Autodesk Fusion 360 part; units mm, degrees
sketch "Sketch3" plane through (0, 0, 0) normal (0, 0, 1) x (1, 0, 0)
  line L0 (10, 15) -> (-10, 15)
  line L1 (-10, 15) -> (-10, -15)
  line L2 (-10, -15) -> (10, -15)
  line L3 (10, -15) -> (10, 15)
  line L4 (10, 15) -> (-10, -15) construction
  line L5 (-10, 15) -> (10, -15) construction
  circle A0 centre (-5.1854, -3.7051) radius 3.5
  circle A1 centre (4.3644, -3.6049) radius 3.5
  circle A2 centre (-5.0469, -11.1711) radius 3.5
  circle A3 centre (4.3207, -10.8626) radius 3.5
  circle A4 centre (-5.1568, 3.7146) radius 3.5
  circle A5 centre (4.2608, 3.6364) radius 3.5
  circle A6 centre (-5.0509, 11.1009) radius 3.5
  circle A7 centre (4.7212, 11.0813) radius 3.5
  dimension "d22" = 20
  dimension "d23" = 30
  dimension "d24" = 7
  dimension "d25" = 7
  dimension "d26" = 7
  dimension "d27" = 7
  dimension "d34" = 7
  dimension "d35" = 7
  dimension "d36" = 7
  dimension "d37" = 7
extrude "Extrude6" add sketch "Sketch3" along normal blind 4
sketch "Sketch5" plane through (0, 0, 4) normal (0, 0, 1) x (-1, 0, 0)
  circle A0 centre (5.1854, 3.7051) radius 3.5
  circle A1 centre (5.0469, 11.1711) radius 3.5
  circle A2 centre (-4.3644, 3.6049) radius 3.5
  circle A3 centre (-4.3207, 10.8626) radius 3.5
  circle A4 centre (5.1568, -3.7146) radius 3.5
  circle A5 centre (-4.2608, -3.6364) radius 3.5
  circle A6 centre (5.0509, -11.1009) radius 3.5
  circle A7 centre (-4.7212, -11.0813) radius 3.5
  line L0 (-10, 15) -> (-10, -15)
  line L1 (-10, -15) -> (10, -15)
  line L2 (10, -15) -> (10, 15)
  line L3 (10, 15) -> (-10, 15)
  line L4 (-10, -15) -> (-8.5, -15)
  line L5 (-8.5, -15) -> (-8.5, -13.5)
  line L6 (-8.5, -13.5) -> (-10, -13.5)
  line L7 (-10, -13.5) -> (-10, -15)
  dimension "d40" = 1.5
  dimension "d41" = 1.5
extrude "Extrude7" cut sketch "Sketch5" against normal blind 4 contours L0 L1 L4 L5 L6 L7
thread "Thread6"
thread "Thread7"
thread "Thread8"
thread "Thread9"
thread "Thread10"
thread "Thread11"
thread "Thread12"
thread "Thread13"
Geometry: final body of the model. Coordinates: model frame, mm. A direction names the side the tool comes from. Give positions to 0.01 mm unless a question says otherwise; leave off trailing zeros. Write each loop counter-clockwise with the first axis right and the second up, starting at its lowest first coordinate (ties: lowest second). Pieces come first, ordered by that corner, then holes. Notation, with made-up numbers: M -1.75,58.5 L 14.25,58.5 A22 ccw 14.25,86.5 Z; hole C 23,86.25 d4. An arc over 180 degrees is marked long. Answer in a Markdown table with one row per item. Add a question column.
(1) Ray query, line 1 (Y direction, x = -7, z = 0.55); line 2 (X direction, y = -3.75, z = 0.6); line 3 (X direction, y = 13, z = 0.65). Return the intervals inside material, ascending.
(2) Section B-B on x = -2.5. Return loops of the section in (y, z).
(3) Reachability of faces 1 (the flat face through (8.5, 14, 2)), 2 (the cylindrical face through (-3.304, -6.656, 1.972)) from +Z, -Z, +X, -X, +Y, -Y: full face, straight path, thin tool, end or side. Return the list, or none.
(4) First-contact query: pin 1 (3 mm diameter, centred on x = -5.5, y = -5.5, fed in from +Z); pin 2 (9 mm diameter, centred on x = 4.26, y = 3.64, fed in from +Z); pin 3 (0.8 mm diameter, centred on y = 14.5, z = 3, fed in from +X); pin 4 (1.6 mm diameter, centred on x = 9.5, z = 1.5, fed in from +Y). Flat tips, straight axial feed; report the tip coordinate or a pass-through.
(5) Section D-D on x = -6.75. Return loops of the section in (y, z), and give its area (3 significant figures).
(6) Section A-A on y = 10.25. Return loops of the section in (x, z), and give its area (3 significant figures).
(7) Section C-C on z = 0.55. State how many separate pieces and enclosed holes the cut face has, and give its area (3 significant figures).
(8) Mould query, pull axis Y, two halves, no side actions, for faces 3 (the cylindrical face through (6.246, -6.556, 1.972)), 4 (the flat face through (-1, 15, 2)), 5 (the flat face through (0, 0, 4)). Classes: +Y half, -Y half, draft (parallel to the pull), parting line (faces both ways), or undercut.
Result set:
| question | item | result |
|---|---|---|
| 1 | line 1 | y = -15 to -14.08, -8.27 to -6.7, -0.71 to 0.74, 6.69 to 8.19, 14.01 to 15 |
| 1 | line 2 | x = -10 to -8.69, -1.69 to 0.87, 7.86 to 10 |
| 1 | line 3 | x = -10 to -7.99, -2.11 to 1.79, 7.65 to 10 |
| 2 | outline | M -15,0 L -13.57,0 L -13.57,4 L -15,4 Z; M -8.77,0 L -5.95,0 L -5.95,4 L -8.77,4 Z; M -1.46,0 L 1.44,0 L 1.44,4 L -1.46,4 Z; M 5.99,0 L 8.7,0 L 8.7,4 L 5.99,4 Z; M 13.5,0 L 15,0 L 15,4 L 13.5,4 Z |
| 3 | face 1 | +Z, -Z, +X, +Y |
| 3 | face 2 | +Z, -Z |
| 4 | pin 1 | passes through |
| 4 | pin 2 | stops at z = 4 |
| 4 | pin 3 | stops at x = 8.5 |
| 4 | pin 4 | stops at y = 13.5 |
| 5 | outline | M -15,0 L -14.23,0 L -14.23,4 L -15,4 Z; M -8.11,0 L -6.84,0 L -6.84,4 L -8.11,4 Z; M -0.57,0 L 0.6,0 L 0.6,4 L -0.57,4 Z; M 6.83,0 L 8.04,0 L 8.04,4 L 6.83,4 Z; M 14.16,0 L 15,0 L 15,4 L 14.16,4 Z |
| 5 | area | 21.1 mm^2 |
| 6 | outline | M -10,0 L -8.45,0 L -8.45,4 L -10,4 Z; M -1.66,0 L 1.32,0 L 1.32,4 L -1.66,4 Z; M 8.12,0 L 10,0 L 10,4 L 8.12,4 Z |
| 6 | area | 25.6 mm^2 |
| 7 | separate pieces | 1 |
| 7 | enclosed holes | 8 |
| 7 | area | 290 mm^2 |
| 8 | face 3 | undercut |
| 8 | face 4 | +Y half |
| 8 | face 5 | draft |
